Geometry: final body of the model. Coordinates: model frame, mm. Face numbers are marked on the shaded views. Coordinates: 2 decimals unless noted, no trailing zeros. Write each loop counter-clockwise with the first axis right and the second up, starting at its lowest first coordinate (ties: lowest second). Pieces come first, ordered by that corner, then holes.
from build123d import *

# Parameters (mm, degrees)
SKETCH1_R                 = 4.2
BOSS_EXTRUDE1_DEPTH       = 3
CUT_EXTRUDE2_DEPTH        = 3
CIRPATTERN1_COUNT         = 12
CIRPATTERN1_COPY_1_DEPTH  = 3
CIRPATTERN1_COPY_2_DEPTH  = 3
CIRPATTERN1_COPY_3_DEPTH  = 3
CIRPATTERN1_COPY_4_DEPTH  = 3
CIRPATTERN1_COPY_5_DEPTH  = 3
CIRPATTERN1_COPY_6_DEPTH  = 3
CIRPATTERN1_COPY_7_DEPTH  = 3
CIRPATTERN1_COPY_8_DEPTH  = 3
CIRPATTERN1_COPY_9_DEPTH  = 3
CIRPATTERN1_COPY_10_DEPTH = 3
CIRPATTERN1_COPY_11_DEPTH = 3


with BuildPart() as part:
    # Sketch1 → Boss-Extrude1 (new body)
    with BuildSketch(Plane(origin=(0, 0, 0), x_dir=(1, 0, 0), z_dir=(0, 1, 0))):
        with Locations(Location((0, 0, 0), (0, 0, 270))):
            Circle(SKETCH1_R)
    extrude(amount=BOSS_EXTRUDE1_DEPTH)

    # Sketch2 → Cut-Extrude2 (cut)
    with BuildSketch(Plane(origin=(0, 3, 0), x_dir=(1, 0, 0), z_dir=(0, 1, 0))):
        with BuildLine():
            Line((-1.108658308, 4.191722636), (0, 5.977827248))
            Line((0, 5.977827248), (0, 2.85))
            ThreePointArc((0, 2.85), (-0.146635628, 2.846225218), (-0.292882823, 2.834910872))
            ThreePointArc((-0.292882823, 2.834910872), (-0.454077223, 3.661639746), (-1.108658308, 4.191722636))
        make_face()
    cut_extrude2 = extrude(amount=-CUT_EXTRUDE2_DEPTH, mode=Mode.SUBTRACT)

    # Mirror2: Cut-Extrude2 across plane
    add(cut_extrude2.mirror(Plane.ZY), mode=Mode.SUBTRACT)

    # CirPattern1: Cut-Extrude2 ×12 about axis
    cirpattern1_axis = Axis((0, 0, 0), (0, 1, 0))
    for i in range(1, CIRPATTERN1_COUNT):
        add(cut_extrude2.rotate(cirpattern1_axis, i * 360 / CIRPATTERN1_COUNT), mode=Mode.SUBTRACT)

    # CirPattern1 copy 1 sketch → CirPattern1 copy 1 (cut)
    with BuildSketch(Plane(origin=(0, 3, 0), x_dir=(-0.8660254037844387, 0, 0.49999999999999994), z_dir=(0, 1, 0))):
        with BuildLine():
            Line((-1.108658308, -4.191722636), (0, -5.977827248))
            Line((0, -5.977827248), (0, -2.85))
            ThreePointArc((0, -2.85), (-0.146635628, -2.846225218), (-0.292882823, -2.834910872))
            ThreePointArc((-0.292882823, -2.834910872), (-0.454077223, -3.661639746), (-1.108658308, -4.191722636))
        make_face()
    extrude(amount=-CIRPATTERN1_COPY_1_DEPTH, mode=Mode.SUBTRACT)

    # CirPattern1 copy 2 sketch → CirPattern1 copy 2 (cut)
    with BuildSketch(Plane(origin=(0, 3, 0), x_dir=(-0.5000000000000001, 0, 0.8660254037844386), z_dir=(0, 1, 0))):
        with BuildLine():
            Line((-1.108658308, -4.191722636), (0, -5.977827248))
            Line((0, -5.977827248), (0, -2.85))
            ThreePointArc((0, -2.85), (-0.146635628, -2.846225218), (-0.292882823, -2.834910872))
            ThreePointArc((-0.292882823, -2.834910872), (-0.454077223, -3.661639746), (-1.108658308, -4.191722636))
        make_face()
    extrude(amount=-CIRPATTERN1_COPY_2_DEPTH, mode=Mode.SUBTRACT)

    # CirPattern1 copy 3 sketch → CirPattern1 copy 3 (cut)
    with BuildSketch(Plane.ZX.offset(3)):
        with BuildLine():
            Line((-1.108658308, -4.191722636), (0, -5.977827248))
            Line((0, -5.977827248), (0, -2.85))
            ThreePointArc((0, -2.85), (-0.146635628, -2.846225218), (-0.292882823, -2.834910872))
            ThreePointArc((-0.292882823, -2.834910872), (-0.454077223, -3.661639746), (-1.108658308, -4.191722636))
        make_face()
    extrude(amount=-CIRPATTERN1_COPY_3_DEPTH, mode=Mode.SUBTRACT)

    # CirPattern1 copy 4 sketch → CirPattern1 copy 4 (cut)
    with BuildSketch(Plane(origin=(0, 3, 0), x_dir=(0.4999999999999998, 0, 0.8660254037844387), z_dir=(0, 1, 0))):
        with BuildLine():
            Line((-1.108658308, -4.191722636), (0, -5.977827248))
            Line((0, -5.977827248), (0, -2.85))
            ThreePointArc((0, -2.85), (-0.146635628, -2.846225218), (-0.292882823, -2.834910872))
            ThreePointArc((-0.292882823, -2.834910872), (-0.454077223, -3.661639746), (-1.108658308, -4.191722636))
        make_face()
    extrude(amount=-CIRPATTERN1_COPY_4_DEPTH, mode=Mode.SUBTRACT)

    # CirPattern1 copy 5 sketch → CirPattern1 copy 5 (cut)
    with BuildSketch(Plane(origin=(0, 3, 0), x_dir=(0.8660254037844387, 0, 0.49999999999999994), z_dir=(0, 1, 0))):
        with BuildLine():
            Line((-1.108658308, -4.191722636), (0, -5.977827248))
            Line((0, -5.977827248), (0, -2.85))
            ThreePointArc((0, -2.85), (-0.146635628, -2.846225218), (-0.292882823, -2.834910872))
            ThreePointArc((-0.292882823, -2.834910872), (-0.454077223, -3.661639746), (-1.108658308, -4.191722636))
        make_face()
    extrude(amount=-CIRPATTERN1_COPY_5_DEPTH, mode=Mode.SUBTRACT)

    # CirPattern1 copy 6 sketch → CirPattern1 copy 6 (cut)
    with BuildSketch(Plane(origin=(0, 3, 0), x_dir=(1, 0, 0), z_dir=(0, 1, 0))):
        with BuildLine():
            Line((-1.108658308, -4.191722636), (0, -5.977827248))
            Line((0, -5.977827248), (0, -2.85))
            ThreePointArc((0, -2.85), (-0.146635628, -2.846225218), (-0.292882823, -2.834910872))
            ThreePointArc((-0.292882823, -2.834910872), (-0.454077223, -3.661639746), (-1.108658308, -4.191722636))
        make_face()
    extrude(amount=-CIRPATTERN1_COPY_6_DEPTH, mode=Mode.SUBTRACT)

    # CirPattern1 copy 7 sketch → CirPattern1 copy 7 (cut)
    with BuildSketch(Plane(origin=(0, 3, 0), x_dir=(0.8660254037844386, 0, -0.5000000000000001), z_dir=(0, 1, 0))):
        with BuildLine():
            Line((-1.108658308, -4.191722636), (0, -5.977827248))
            Line((0, -5.977827248), (0, -2.85))
            ThreePointArc((0, -2.85), (-0.146635628, -2.846225218), (-0.292882823, -2.834910872))
            ThreePointArc((-0.292882823, -2.834910872), (-0.454077223, -3.661639746), (-1.108658308, -4.191722636))
        make_face()
    extrude(amount=-CIRPATTERN1_COPY_7_DEPTH, mode=Mode.SUBTRACT)

    # CirPattern1 copy 8 sketch → CirPattern1 copy 8 (cut)
    with BuildSketch(Plane(origin=(0, 3, 0), x_dir=(0.5000000000000004, 0, -0.8660254037844384), z_dir=(0, 1, 0))):
        with BuildLine():
            Line((-1.108658308, -4.191722636), (0, -5.977827248))
            Line((0, -5.977827248), (0, -2.85))
            ThreePointArc((0, -2.85), (-0.146635628, -2.846225218), (-0.292882823, -2.834910872))
            ThreePointArc((-0.292882823, -2.834910872), (-0.454077223, -3.661639746), (-1.108658308, -4.191722636))
        make_face()
    extrude(amount=-CIRPATTERN1_COPY_8_DEPTH, mode=Mode.SUBTRACT)

    # CirPattern1 copy 9 sketch → CirPattern1 copy 9 (cut)
    with BuildSketch(Plane(origin=(0, 3, 0), x_dir=(0, 0, -1), z_dir=(0, 1, 0))):
        with BuildLine():
            Line((-1.108658308, -4.191722636), (0, -5.977827248))
            Line((0, -5.977827248), (0, -2.85))
            ThreePointArc((0, -2.85), (-0.146635628, -2.846225218), (-0.292882823, -2.834910872))
            ThreePointArc((-0.292882823, -2.834910872), (-0.454077223, -3.661639746), (-1.108658308, -4.191722636))
        make_face()
    extrude(amount=-CIRPATTERN1_COPY_9_DEPTH, mode=Mode.SUBTRACT)

    # CirPattern1 copy 10 sketch → CirPattern1 copy 10 (cut)
    with BuildSketch(Plane(origin=(0, 3, 0), x_dir=(-0.5000000000000001, 0, -0.8660254037844386), z_dir=(0, 1, 0))):
        with BuildLine():
            Line((-1.108658308, -4.191722636), (0, -5.977827248))
            Line((0, -5.977827248), (0, -2.85))
            ThreePointArc((0, -2.85), (-0.146635628, -2.846225218), (-0.292882823, -2.834910872))
            ThreePointArc((-0.292882823, -2.834910872), (-0.454077223, -3.661639746), (-1.108658308, -4.191722636))
        make_face()
    extrude(amount=-CIRPATTERN1_COPY_10_DEPTH, mode=Mode.SUBTRACT)

    # CirPattern1 copy 11 sketch → CirPattern1 copy 11 (cut)
    with BuildSketch(Plane(origin=(0, 3, 0), x_dir=(-0.8660254037844384, 0, -0.5000000000000004), z_dir=(0, 1, 0))):
        with BuildLine():
            Line((-1.108658308, -4.191722636), (0, -5.977827248))
            Line((0, -5.977827248), (0, -2.85))
            ThreePointArc((0, -2.85), (-0.146635628, -2.846225218), (-0.292882823, -2.834910872))
            ThreePointArc((-0.292882823, -2.834910872), (-0.454077223, -3.661639746), (-1.108658308, -4.191722636))
        make_face()
    extrude(amount=-CIRPATTERN1_COPY_11_DEPTH, mode=Mode.SUBTRACT)


solid = part.part
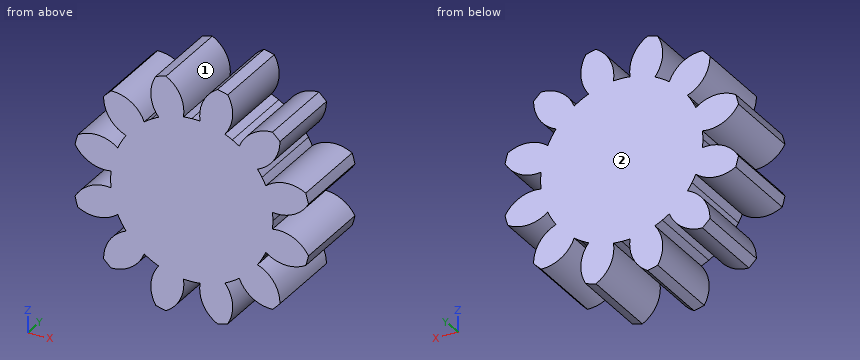
Item 1: Section C-C, the plane x = -3. Output: boundary loops of the cut face in (y, z), plus the area to 3 significant figures.
Derived:
outline: (0, -2.94) - (3, -2.94) - (3, -2.34) - (0, -2.34) - close; (0, -1.38) - (3, -1.38) - (3, -0.28) - (0, -0.28) - close; (0, 0.28) - (3, 0.28) - (3, 1.38) - (0, 1.38) - close; (0, 2.34) - (3, 2.34) - (3, 2.94) - (0, 2.94) - close
area: 10.2 mm2
Item 2: Section A-A, the plane x = 3.5. Output: boundary loops of the cut face in (y, z), plus the area to 3 significant figures.
Derived:
outline: (0, -1.43) - (3, -1.43) - (3, -0.37) - (0, -0.37) - close; (0, 0.37) - (3, 0.37) - (3, 1.43) - (0, 1.43) - close
area: 6.35 mm2
Item 3: Section D-D, the plane x = -0.75. Output: boundary loops of the cut face in (y, z).
Derived:
outline: (0, -4) - (3, -4) - (3, 4) - (0, 4) - close
Item 4: Material intervals for probe 1 along Z at (x, y) = (2.75, 2.9); probe 2 along X at (y, z) = (2.1, 2.5), sorted ascending.
Derived:
probe 1: z = -3.1 to -1.96, -1.27 to 1.27, 1.96 to 3.1
probe 2: x = -3.06 to -1.76, -1.37 to 1.37, 1.76 to 3.06
Item 5: Pull-direction query (X, two-part tool) for the marked faces 1 and 2; classes: released by +X, released by -X, zero draft, split by the parting line, or undercut.
Derived:
face 1: undercut
face 2: zero draft
Item 6: Section B-B, the plane z = -3.25. Output: boundary loops of the cut face in (x, y).
Derived:
outline: (-1.43, 0) - (-0.3, 0) - (-0.3, 3) - (-1.43, 3) - close; (0.3, 0) - (1.43, 0) - (1.43, 3) - (0.3, 3) - close
